from build123d import *

# Parameters (mm, degrees)
SKETCH1_W             = 81.5848
SKETCH1_H             = 51.943
BOSS_EXTRUDE1_DEPTH   = 3.81
SKETCH2_W             = 63.5
SKETCH2_H             = 5.08
BOSS_EXTRUDE2_DEPTH   = 20.1168
SKETCH3_W             = 81.5848
SKETCH3_H             = 5.08
BOSS_EXTRUDE3_DEPTH   = 3.175
SKETCH4_W             = 63.5
SKETCH4_H             = 5.08
BOSS_EXTRUDE4_DEPTH   = 10.033
SKETCH6_W             = 3.175
SKETCH6_H             = 21.59
BOSS_EXTRUDE5_DEPTH   = 8.89
FILLET1_R             = 6.35
SKETCH7_W             = 9.0424
SKETCH7_H             = 5.08
BOSS_EXTRUDE6_DEPTH   = 5.08
FILLET2_R             = 6.35
FILLET3_R             = 6.35
SKETCH8_W             = 1.27
SKETCH8_H             = 41.783
BOSS_EXTRUDE7_DEPTH   = 3.175
F_6_CLEARANCE_HOLE1_D = 3.7973


with BuildPart() as part:
    # Sketch1 → Boss-Extrude1 (new body)
    with BuildSketch(Plane(origin=(0, 0, 0), x_dir=(1, 0, 0), z_dir=(0, 1, 0))):
        Rectangle(SKETCH1_W, SKETCH1_H)
    extrude(amount=BOSS_EXTRUDE1_DEPTH)

    # Sketch2 → Boss-Extrude2 (add)
    with BuildSketch(Plane.XZ):
        with Locations((0, 23.4315)):
            Rectangle(SKETCH2_W, SKETCH2_H)
    extrude(amount=BOSS_EXTRUDE2_DEPTH)

    # Sketch3 → Boss-Extrude3 (add)
    with BuildSketch(Plane.XZ):
        with Locations((0, -23.4315)):
            Rectangle(SKETCH3_W, SKETCH3_H)
    extrude(amount=BOSS_EXTRUDE3_DEPTH)

    # Sketch4 → Boss-Extrude4 (add)
    with BuildSketch(Plane.XY.offset(25.9715)):
        with Locations((0, -17.5768)):
            Rectangle(SKETCH4_W, SKETCH4_H)
    extrude(amount=BOSS_EXTRUDE4_DEPTH)

    # Sketch6 → Boss-Extrude5 (add)
    with BuildSketch(Plane(origin=(0, 3.81, 0), x_dir=(1, 0, 0), z_dir=(0, 1, 0))):
        with Locations((-42.3799, -15.1765)):
            Rectangle(SKETCH6_W, SKETCH6_H)
        with Locations((42.3799, -15.1765)):
            Rectangle(SKETCH6_W, SKETCH6_H)
    extrude(amount=-BOSS_EXTRUDE5_DEPTH)

    # Fillet1
    fillet1_edges = [part.edges().sort_by_distance(p)[0] for p in [
        (0, 3.81, -25.9715),
    ]]
    fillet(fillet1_edges, radius=FILLET1_R)

    # Sketch7 → Boss-Extrude6 (add)
    with BuildSketch(Plane.XY.offset(25.9715)):
        with Locations((36.2712, -2.54)):
            Rectangle(SKETCH7_W, SKETCH7_H)
        with Locations((-36.2712, -2.54)):
            Rectangle(SKETCH7_W, SKETCH7_H)
    extrude(amount=-BOSS_EXTRUDE6_DEPTH)

    # Fillet2
    fillet2_edges = [part.edges().sort_by_distance(p)[0] for p in [
        (-31.75, -5.08, 23.4315),
        (31.75, -5.08, 23.4315),
    ]]
    fillet(fillet2_edges, radius=FILLET2_R)

    # Fillet3
    fillet3_edges = [part.edges().sort_by_distance(p)[0] for p in [
        (0, 3.81, 25.9715),
    ]]
    fillet(fillet3_edges, radius=FILLET3_R)

    # Sketch8 → Boss-Extrude7 (add)
    with BuildSketch(Plane.XZ):
        Rectangle(SKETCH8_W, SKETCH8_H)
    extrude(amount=BOSS_EXTRUDE7_DEPTH)

    # #6 Clearance Hole1 (through all)
    with Locations(Plane(origin=(21.59, -15.0368, 30.988), x_dir=(0, 0, 1), z_dir=(0, 1, 0))):
        with Locations((0, 0), (0, -43.18), (0, -21.59)):
            Hole(F_6_CLEARANCE_HOLE1_D / 2)


solid = part.part
Check sheet for the modelled part. Datum: model origin and axes. Units: mm. A direction names the side the tool comes from. Round coordinates to 2 decimals unless told otherwise and drop trailing zeros. Loops run counter-clockwise (first coordinate to the right, second up) from the corner with the lowest first, then second, coordinate; pieces in that order, holes last. Notation, with made-up numbers: (-26, 65.25) - (17, 65.25) arc R25 ccw to (17, 102.25) - close; hole circle Ø7 at (-27, -20.75). An arc over 180 degrees is marked (long way). Answer as CSV lines item,"result". Start each with the question number.
Item 1: Section check D-D (z = 5.5). Record the boundary of the cut face in (x, y) (3 decimals).
Item 2: Section check C-C (z = 31). Record the boundary of the cut face in (x, y).
Item 3: Depth check by flat-ended pin: P1, Ø20, axis at x = -22.5, z = 4, coming from the -Y side; P2, Ø5.5, axis at y = 2, z = -17.5, coming from the -X side; P3, Ø1, axis at x = -42, y = 0, coming from the -Z side; P4, Ø2.5, axis at x = -21.59, z = 30.988, coming from the -Y side. Enter the tip coordinate at first touch or a pass-through.
Item 4: Release check for a two-part mould opening along X. For faces 1 (the flat face through (0, -20.117, 28)), 2 (the cylindrical face through (-22.75, -17.61, 32.49)), 3 (the flat face through (43.967, -1, 15)) record: +X half, -X half, draft (parallel to the pull), parting line (faces both ways), or undercut.
Item 5: Scan lines: line 1 (X direction, y = -2.5, z = 13) (3 decimals); line 2 (Z direction, x = -36, y = -2.25); line 3 (Y direction, x = -13, z = -2). Record each from-to range of solid material in increasing order. Write a range as [from, to].
Item 6: Section check A-A (z = -11). Record the boundary of the cut face in (x, y) (3 decimals).
Item 7: Set-up check for faces 4 (the flat face through (31.75, -17, 27)), 5 (the flat face through (-40.792, 1, -11)), 6 (the flat face through (-21, -2, -20.892)), 7 (the flat face through (40.792, 1, -11)), 8 (the flat face through (-0.635, -2, 0)): record each of +Z, -Z, +X, -X, +Y, -Y from which the full face is reachable in a straight line by a thin tool's end or side.
Report:
1,outline,"(-43.967, -5.08) - (-40.792, -5.08) - (-40.792, 0) - (-0.635, 0) - (-0.635, -3.175) - (0.635, -3.175) - (0.635, 0) - (40.792, 0) - (40.792, -5.08) - (43.967, -5.08) - (43.967, 3.81) - (-43.967, 3.81) - close"
2,outline,"(-31.75, -20.12) - (-23.49, -20.12) - (-23.49, -15.04) - (-31.75, -15.04) - close; (-19.69, -20.12) - (-1.9, -20.12) - (-1.9, -15.04) - (-19.69, -15.04) - close; (1.9, -20.12) - (19.69, -20.12) - (19.69, -15.04) - (1.9, -15.04) - close; (23.49, -20.12) - (31.75, -20.12) - (31.75, -15.04) - (23.49, -15.04) - close"
3,P1,"stops at y = 0"
3,P2,"stops at x = -40.79"
3,P3,"stops at z = 4.38"
3,P4,"passes through"
4,face 1,"draft"
4,face 2,"undercut"
4,face 3,"+X half"
5,line 1,"x = [-43.967, -40.792], [-0.635, 0.635], [40.792, 43.967]"
5,line 2,"z = [-25.96, -20.89], [20.89, 25.96]"
5,line 3,"y = [0, 3.81]"
6,outline,"(-40.792, 0) - (-0.635, 0) - (-0.635, -3.175) - (0.635, -3.175) - (0.635, 0) - (40.792, 0) - (40.792, 3.81) - (-40.792, 3.81) - close"
7,face 4,"+Z, -Z, +X, -Y"
7,face 5,"-Z, -X, +Y, -Y"
7,face 6,"-X, -Y"
7,face 7,"-Z, +X, +Y, -Y"
7,face 8,"-Y"
